Input: part model. Units: mm. Frame: model coordinates. Face numbers are marked on the shaded views. A direction names the side the tool comes from. Coordinates: 2 decimals unless noted, no trailing zeros. Loops run counter-clockwise (first coordinate to the right, second up) from the corner with the lowest first, then second, coordinate; pieces in that order, holes last. Notation, with made-up numbers: (-8.75, -5) -> (-1.75, -5) arc R17 ccw to (-1.75, 8) -> close; hole circle Ø9 at (-9.75, 48.5). An arc over 180 degrees is marked (long way). Put each result on its own line as item: value. Start each with the question number.
1) Pull-direction query (X, two-part tool) for the marked faces 3, 4 and 5; classes: pulls with the +X half, pulls with the -X half, needs draft (parallel to the pull), parting line crosses it, or undercut.
2) Material intervals for L1, parallel to Y at x = 21.5, z = 1.45; L2, parallel to X at y = 0.5, z = 4.75; L3, parallel to X at y = 17.5, z = 3.8, sorted ascending.
3) Cut plane A-A (y = 5.5). Return the cut outline in (x, z), plus the area to 3 significant figures.
4) Cut plane B-B (x = -4.5). Return the cut outline in (y, z).
5) Set-up query: the marked faces 1 and 2. Return all of +Z, -Z, +X, -X, +Y, -Y with unobstructed straight access to the full face (end or side cutting, diameter ignored); none if empty.
from build123d import *

# Parameters (mm, degrees)
F1_DEPTH = 5
F2_W     = 34.4714387385
F2_H     = 10
F2_W_2   = 10
F3_DEPTH = 5


# Not quite as in the source:
# - ends of sketch curves that miss each other by under 0.0002 mm in the source are joined


with BuildPart() as f1:
    # F0 (on Top) → F1 (new body)
    with BuildSketch(Plane.XY):
        with BuildLine():
            Line((0, 29.2999204248), (0, 0))
            Line((0, 0), (34.4714387385, 0))
            Line((34.4714387385, 0), (34.4714387385, 16.3473710418))
            ThreePointArc((34.4714387385, 16.3473710418), (32.5790927131, 15.1300794804), (32.2559916738, 17.3568210333))
            ThreePointArc((32.2559916738, 17.3568210333), (15.182844974, 14.8438668457), (5.7578901922, 29.2999210911))
            ThreePointArc((5.7578901922, 29.2999210911), (2.8789043427, 26.4210160822), (0, 29.2999204248))
        make_face()
        with BuildLine():
            ThreePointArc((5.7577396052, 29.3198639813), (2.8689325046, 32.1788074974), (0, 29.2999204248))
            ThreePointArc((0, 29.2999204248), (2.8789043427, 26.4210160822), (5.7578086853, 29.2999204248))
            ThreePointArc((5.7578086853, 29.2999204248), (5.7578117914, 29.3098925127), (5.7577396052, 29.3198639813))
        make_face()
        with BuildLine():
            ThreePointArc((32.2559916738, 17.3568210333), (32.5790927131, 15.1300794804), (34.4714387385, 16.3473710418))
            ThreePointArc((34.4714387385, 16.3473710418), (33.6883902233, 17.5646626032), (32.2559916738, 17.3568210333))
        make_face()
    extrude(amount=F1_DEPTH)

    # F2 (on face) → F3 (join)
    with BuildSketch(Plane.XY.offset(5)):
        with BuildLine():
            Line((0, 0), (34.4714387385, 0))
            Line((34.4714387385, 0), (34.4714387385, 16.3473710418))
            ThreePointArc((34.4714387385, 16.3473710418), (33.6883902233, 17.5646626032), (32.2559916738, 17.3568210333))
            ThreePointArc((32.2559916738, 17.3568210333), (15.182844974, 14.8438668457), (5.7578901922, 29.2999210911))
            ThreePointArc((5.7578901922, 29.2999210911), (5.757811792, 29.3098923335), (5.7577396052, 29.3198639813))
            ThreePointArc((5.7577396052, 29.3198639813), (2.8689325046, 32.1788074974), (0, 29.2999204248))
            Line((0, 29.2999204248), (0, 25.4882741719))
            Line((0, 25.4882741719), (0, 0))
        make_face()
        with Locations((17.2357193692, -5)):
            Rectangle(F2_W, F2_H)
        with Locations((-5, -5)):
            Rectangle(F2_W_2, F2_H)
        with Locations((-5, -5)):
            Rectangle(F2_W_2, F2_H)
    extrude(amount=-F3_DEPTH)


solid = f1.part
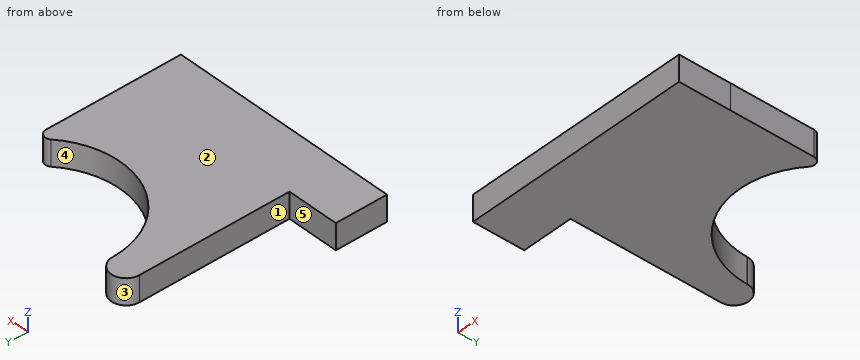
Results found:
1. face 3: parting line crosses it
1. face 4: undercut
1. face 5: needs draft
2. L1: y = -10 to 13.43
2. L2: x = 0 to 34.47
2. L3: x = 0 to 11.1, 32.45 to 33.81
3. outline: (0, 0) -> (34.47, 0) -> (34.47, 5) -> (0, 5) -> close
3. area: 172 mm2
4. outline: (-10, 0) -> (0, 0) -> (0, 5) -> (-10, 5) -> close
5. face 1: +Z, -Z, -X, +Y
5. face 2: +Z, +X, -X, +Y, -Y
